The model under review builds one solid part; all positions refer to its coordinate system, in mm. A direction names the side the tool comes from. Round coordinates to 2 decimals unless told otherwise and drop trailing zeros. Order: outer loops, then holes, each group sorted by start corner. A loop starts at its lowest first (then second) coordinate and runs counter-clockwise, first axis right, second up. Notation, with made-up numbers: M 38,6.5 L 74,6.5 A15 cw 74,21.5 Z; hole C -22,25 d1. An arc over 180 degrees is marked long. Answer as CSV lines item,"result". Start each with the question number.
from build123d import *

# Parameters (mm, degrees)
F0_R     = 16.7
F1_DEPTH = 23
F2_T     = -2.5
F3_R     = 20.65
F3_R_2   = 16.7
F4_DEPTH = 12
F5_R     = 12.7
F6_DEPTH = 17.5
F7_T     = -2.5
F8_R     = 37.5
F8_R_2   = 12.7
F8_R_3   = 10.2
F9_DEPTH = 3.5


with BuildPart() as f1:
    # F0 (on Top) → F1 (new body)
    with BuildSketch(Plane.XY):
        Circle(F0_R)
    extrude(amount=F1_DEPTH)

    # F2
    f2_openings = [f1.faces().sort_by_distance(p)[0] for p in [
        (0, 0, 0),
    ]]
    offset(amount=F2_T, openings=f2_openings)

    # F3 (on face) → F4 (join)
    with BuildSketch(Plane.XY.offset(23)):
        Circle(F3_R)
        Circle(F3_R_2, mode=Mode.SUBTRACT)
        Circle(F3_R_2)
    extrude(amount=F4_DEPTH)

    # F5 (on face) → F6 (join)
    with BuildSketch(Plane.XY.offset(35)):
        Circle(F5_R)
    extrude(amount=F6_DEPTH)

    # F7
    f7_openings = [f1.faces().sort_by_distance(p)[0] for p in [
        (0, 0, 52.5),
    ]]
    offset(amount=F7_T, openings=f7_openings, kind=Kind.INTERSECTION)

    # F8 (on face) → F9 (join)
    with BuildSketch(Plane.XY.offset(52.5)):
        Circle(F8_R)
        Circle(F8_R_2, mode=Mode.SUBTRACT)
        Circle(F8_R_2)
        Circle(F8_R_3, mode=Mode.SUBTRACT)
        Circle(F8_R_3)
    extrude(amount=F9_DEPTH)


solid = f1.part
Item 1: Wall thickness on probe 1 along Z at (x, y) = (2, 18); probe 2 along Z at (x, y) = (-1, 16); probe 3 along Y at (x, z) = (0, 14): over which ranges is each line inside the solid? List them lowest first. Write a range as [from, to].
Item 2: Consider section C-C (z = 37). State the section outline as (x, y) points, and give its area (3 significant figures).
Item 3: Consider section D-D (z = 22). State the section outline as (x, y) points.
Item 4: Tool access review of faces 4 (the cylindrical face through (-4.88, 37.18, 54.23)), 5 (the flat face through (17, 0, 23)), 6 (the cylindrical face through (17.312, 5.452, 28.951)): name each direction out of +Z, -Z, +X, -X, +Y, -Y from which nothing blocks a thin tool from reaching the whole face with its end or side.
Item 5: For pin 1 (22.5 mm diameter, centred on x = 4.5, y = 3, fed in from -Z); pin 2 (10 mm diameter, centred on x = 26, y = 18.5, fed in from -Z); pin 3 (4 mm diameter, centred on y = -9.5, z = 45.5, fed in from +X); pin 4 (1 mm diameter, centred on y = 13, z = 26, fed in from +X), all flat-tipped, find the tip position at first contact; note any pin that passes through.
Item 6: The part is to be moulded in two halves that separate along Y. For faces 1 (the cylindrical face through (-1.85, 14.08, 10.11)), 2 (the flat face through (-8, -12, 0)), 3 (the cylindrical face through (-2.75, -12.4, 43.63)), say which applies: +Y half, -Y half, draft (parallel to the pull), parting line (faces both ways), or undercut.
Reported:
1,probe 1,"z = [23, 25.5], [32.5, 35], [52.5, 56]"
1,probe 2,"z = [0, 25.5], [32.5, 35], [52.5, 56]"
1,probe 3,"y = [-16.7, -14.2], [14.2, 16.7]"
2,outline,"C 0,0 d25.4; hole C 0,0 d20.4"
2,area,"180 mm²"
3,outline,"C 0,0 d33.4"
4,face 4,"+Z, -Z"
4,face 5,"-Z"
4,face 6,"none"
5,pin 1,"stops at z = 0"
5,pin 2,"stops at z = 52.5"
5,pin 3,"stops at x = 10.25"
5,pin 4,"stops at x = 16.44"
6,face 1,"undercut"
6,face 2,"draft"
6,face 3,"parting line"
